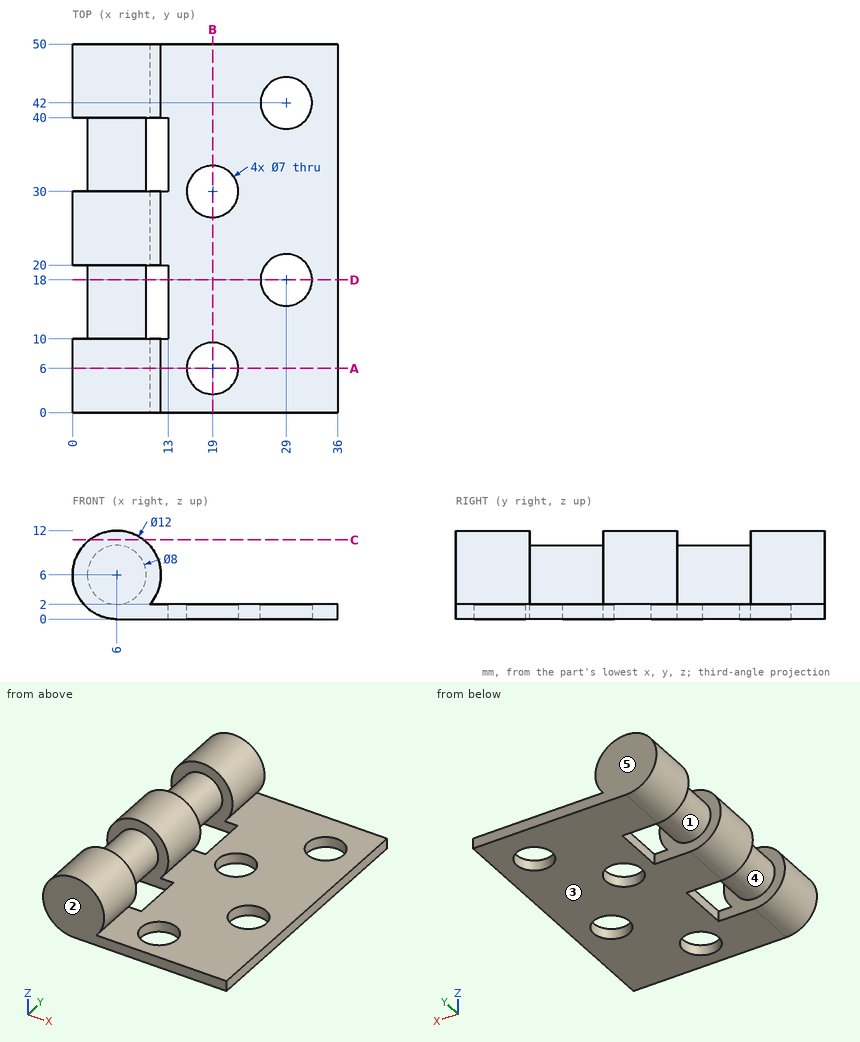
Could you check a few things on this drawing? It's one solid part, dimensions in mm from its lowest x, y, z. A direction names the side the tool comes from. Coordinates: 2 decimals unless noted, no trailing zeros. Order: outer loops, then holes, each group sorted by start corner. A loop starts at its lowest first (then second) coordinate and runs counter-clockwise, first axis right, second up. Notation, with made-up numbers: (53, 88.25) -> (109, 88.25) arc R28 ccw to (109, 127.25) -> close; hole circle Ø1 at (87, 25.25). An arc over 180 degrees is marked (long way). Answer in a Markdown table with one row per item.
(1) Please list where these lines run through material, in increasing order: probe 1 along Y at (x, z) = (29, 0.85); probe 2 along Y at (x, z) = (10, 4.25); probe 3 along Z at (x, y) = (32.5, 18.5).
Answer key:
| item | result |
|---|---|
| probe 1 | 0 to 14.5, 21.5 to 38.5, 45.5 to 50 |
| probe 2 | 0 to 10, 20 to 30, 40 to 50 |
| probe 3 | 0 to 2 |
(2) I want a section at D-D on y = 18. List the corners of the cut face in (x, z) for me, then the cut area to 3 significant figures.
Answer key:
| item | result |
|---|---|
| outline | circle Ø8 at (6, 6); (13, 0) -> (25.5, 0) -> (25.5, 2) -> (13, 2) -> close; (32.5, 0) -> (36, 0) -> (36, 2) -> (32.5, 2) -> close |
| area | 82.3 mm^2 |
(3) Thinking about a two-plate mould opening in Y: for the marked faces 3, 4 and 5, which applies, +Y half, -Y half, draft (parallel to the pull), parting line (faces both ways), or undercut?
Answer key:
| item | result |
|---|---|
| face 3 | draft |
| face 4 | undercut |
| face 5 | +Y half |
(4) I want a section at C-C on z = 10.75. List the corners of the cut face in (x, y) for me.
Answer key:
| item | result |
|---|---|
| outline | (2.33, 0) -> (9.67, 0) -> (9.67, 10) -> (2.33, 10) -> close; (2.33, 20) -> (9.67, 20) -> (9.67, 30) -> (2.33, 30) -> close; (2.33, 40) -> (9.67, 40) -> (9.67, 50) -> (2.33, 50) -> close |
(5) Will these pins go through, and if not, where does the flat tip stop? pin 1 Ø4 at (x, y) = (29, 42) entering from +Z; pin 2 Ø1.6 at (y, z) = (33.5, 1) entering from -X; pin 3 Ø6 at (x, z) = (18.5, 3) entering from +Y; pin 4 Ø1.6 at (y, z) = (17, 1.5) entering from -X.
Answer key:
| item | result |
|---|---|
| pin 1 | through |
| pin 2 | x = 13 |
| pin 3 | y = 50 |
| pin 4 | x = 4.48 |
(6) On a 3-axis mill with a long thin cutter (end or side, diameter ignored), from which of +Z, -Z, +X, -X, +Y, -Y can I reach the whole of each face in a straight line? I mean the marked faces 1 and 2. Say none if no direction works.
Answer key:
| item | result |
|---|---|
| face 1 | none |
| face 2 | +Z, -Z, +X, -X, -Y |
(7) I want a section at B-B on x = 19. List the corners of the cut face in (y, z) for me, then the cut area to 3 significant figures.
Answer key:
| item | result |
|---|---|
| outline | (0, 0) -> (2.5, 0) -> (2.5, 2) -> (0, 2) -> close; (9.5, 0) -> (26.5, 0) -> (26.5, 2) -> (9.5, 2) -> close; (33.5, 0) -> (50, 0) -> (50, 2) -> (33.5, 2) -> close |
| area | 72.0 mm^2 |
(8) I want a section at A-A on y = 6. List the corners of the cut face in (x, z) for me, then the cut area to 3 significant figures.
Answer key:
| item | result |
|---|---|
| outline | (6, 0) -> (15.5, 0) -> (15.5, 2) -> (10.47, 2) arc R6 ccw (long way) to start; (22.5, 0) -> (36, 0) -> (36, 2) -> (22.5, 2) -> close |
| area | 153 mm^2 |
